from build123d import *

# Parameters (mm, degrees)
F0_W     = 99.320174
F0_H     = 83.844102
F1_DEPTH = 25.4
F2_R     = 19.095077
F3_DEPTH = 25.4
F5_DEPTH = 44.35832


with BuildPart() as f1:
    # F0 (on Top) → F1 (new body)
    with BuildSketch(Plane.XY):
        Rectangle(F0_W, F0_H)
    extrude(amount=F1_DEPTH)

    # F2 (on face) → F3 (join)
    with BuildSketch(Plane.XY.offset(25.4)):
        Circle(F2_R)
    extrude(amount=F3_DEPTH)

    # F4 (on Front) → F5 (cut, symmetric)
    with BuildSketch(Plane.XZ):
        Polygon((21.894151, 53.422578), (-26.067015, 53.422578), (21.894151, 31.12971), align=None)
    extrude(amount=F5_DEPTH, both=True, mode=Mode.SUBTRACT)


solid = f1.part
Input: part model. Units: mm. Frame: model coordinates. A direction names the side the tool comes from. Give positions to 0.01 mm unless a question says otherwise; leave off trailing zeros. Write each loop counter-clockwise with the first axis right and the second up, starting at its lowest first coordinate (ties: lowest second). Pieces come first, ordered by that corner, then holes. Notation, with made-up numbers: M 84.5,19.25 L 112.5,19.25 A22 ccw 112.5,51.25 Z; hole C 33.5,22.5 d7. An arc over 180 degrees is marked long. Use one line per item in the form item = value.
1. Cut plane D-D on y = 34. Return loops of the section in (x, z).
Outcome:
outline = M -49.66,0 L 49.66,0 L 49.66,25.4 L -49.66,25.4 Z
2. Reachability of faces 1 (the face through (-19.077, 0.84, 35.004)), 2 (the face through (49.66, -1, 13)) from +Z, -Z, +X, -X, +Y, -Y: full face, straight path, thin tool, end or side. Return the list, or none.
Outcome:
face_1 = +Z
face_2 = +Z, -Z, +X, +Y, -Y
3. Cut plane A-A on y = 0. Return loops of the section in (x, z).
Outcome:
outline = M -49.66,0 L 49.66,0 L 49.66,25.4 L 19.1,25.4 L 19.1,32.43 L -19.1,50.18 L -19.1,25.4 L -49.66,25.4 Z
4. First-contact query: P1, Ø4, axis at x = -15.5, z = 42, coming from the +Y side; P2, Ø3, axis at x = 23.5, y = 4.5, coming from the +Z side; P3, Ø2, axis at x = -10, z = 38.5, coming from the -Y side. Flat tips, straight axial feed; report the tip coordinate or a pass-through.
Outcome:
P1 = 13.5
P2 = 25.4
P3 = -16.84
5. Cut plane C-C on z = 30. Return loops of the section in (x, y), and give its area (3 significant figures).
Outcome:
outline = C 0,0 d38.19
area = 1,150 mm²
6. Cut plane B-B on x = 0. Return loops of the section in (y, z), and give its area (3 significant figures).
Outcome:
outline = M -41.92,0 L 41.92,0 L 41.92,25.4 L 19.1,25.4 L 19.1,41.31 L -19.1,41.31 L -19.1,25.4 L -41.92,25.4 Z
area = 2,740 mm²
7. Ray query, L1, parallel to Z at x = -18.5, y = 12.5; L2, parallel to X at y = -12, z = 43.5; L3, parallel to X at y = 10, z = 45. Return the intervals inside material, ascending.
Outcome:
L1 = 0 to 25.4
L2 = -14.85 to -4.72
L3 = -16.27 to -7.95
